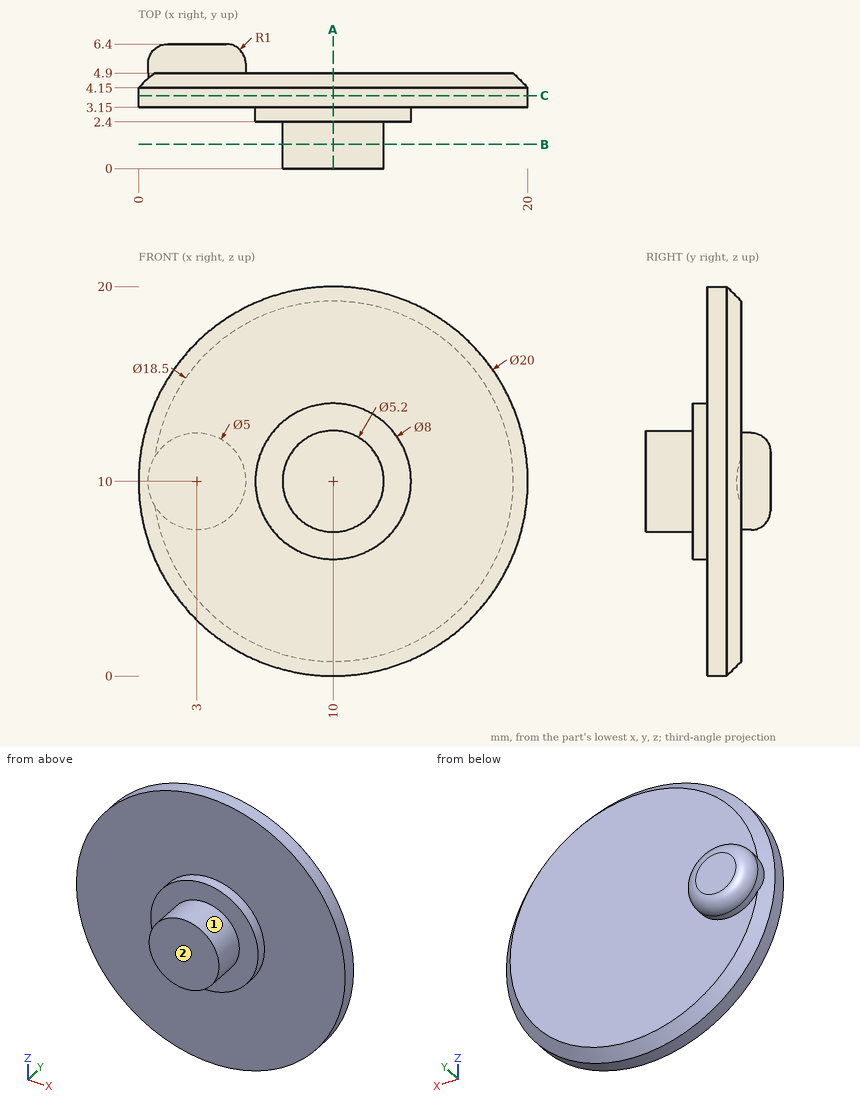
Job drawing, mm, ordinate dimensions from the low corner. One solid piece. A direction names the side the tool comes from. Give positions to 0.01 mm unless a question says otherwise; leave off trailing zeros. Order: outer loops, then holes, each group sorted by start corner. A loop starts at its lowest first (then second) coordinate and runs counter-clockwise, first axis right, second up. Notation, with made-up numbers: (75.5, 24.5) -> (113.5, 24.5) arc R21 ccw to (113.5, 62.5) -> close; hole circle Ø1 at (15.25, -27). An arc over 180 degrees is marked (long way). Return JSON: item names as keys, results as strings.
Q1. Drill centre lines: line 1 (Y direction, x = 14.75, z = 15.5); line 2 (Z direction, x = 10, y = 2.25); line 3 (Z direction, x = 3.5, y = 3.25). Where is each one in solid material? Low to high.
Working result:
{"line 1": "3.15 to 4.9", "line 2": "7.4 to 12.6", "line 3": "2.4 to 17.6"}
Q2. Saw through at C-C (y = 3.75). Write the cut outline in (x, z), then the cut area to 3 significant figures.
Working result:
{"outline": "circle Ø20 at (10, 10)", "area": "314 mm²"}
Q3. Flat gauge pins, fed straight in: pin 1 (4 mm diameter, centred on x = 8.5, z = 6.5, fed in from +Y); pin 2 (1.5 mm diameter, centred on x = 17.5, y = 3, fed in from +Z); pin 3 (8 mm diameter, centred on x = 15.5, z = 17.5, fed in from -Y). Where does each tip first touch, or does it go through?
Working result:
{"pin 1": "y = 4.9", "pin 2": "z = 17.36", "pin 3": "y = 3.15"}
Q4. Saw through at A-A (x = 10). Write the cut outline in (y, z).
Working result:
{"outline": "(0, 7.4) -> (2.4, 7.4) -> (2.4, 6) -> (3.15, 6) -> (3.15, 0) -> (4.15, 0) -> (4.9, 0.75) -> (4.9, 19.25) -> (4.15, 20) -> (3.15, 20) -> (3.15, 14) -> (2.4, 14) -> (2.4, 12.6) -> (0, 12.6) -> close"}
Q5. Saw through at B-B (y = 1.25). Write the cut outline in (x, z).
Working result:
{"outline": "circle Ø5.2 at (10, 10)"}
Q6. Which spindle directions (+Z, -Z, +X, -X, +Y, -Y) get a long thin tool onto all of the face, cutting with end or side? Do the marked faces 1 and 2. Say none if no direction does.
Working result:
{"face 1": "-Y", "face 2": "+Z, -Z, +X, -X, -Y"}
